Can you work these out from the drawing? Everything is in mm from the part's minimum corner. A direction names the side the tool comes from. Coordinates: 2 decimals unless noted, no trailing zeros. Loops run counter-clockwise (first coordinate to the right, second up) from the corner with the lowest first, then second, coordinate; pieces in that order, holes last. Notation, with made-up numbers: (41, -28) -> (63, -28) arc R27 cw to (63, 7) -> close; hole circle Ø8 at (-9.5, -9.5). An arc over 180 degrees is marked (long way). Use one line per item in the form item = value. Start each with the question number.
(1) Imagine slicing it at D-D (x = 37.5). List the corners of the cut face in (y, z) for me.
(2) Imagine slicing it at B-B (x = 47). List the corners of the cut face in (y, z) for me, plus the area to 3 significant figures.
(3) I need wall thicknesses on line 1 (Z direction, x = 37.5, y = 1.6); line 2 (Y direction, x = 37, z = 9.75); line 3 (Z direction, x = 40.5, y = 69). Which ranges of each line are inside material? Lowest first, please. Write a range as [from, to].
(4) On a 3-axis mill with a long thin cutter (end or side, diameter ignored), from which of +Z, -Z, +X, -X, +Y, -Y can I reach the whole of each face in a straight line? I mean the marked faces 1 and 2. Say none if no direction works.
(5) Imagine slicing it at A-A (z = 16.5). State how many separate pieces and enclosed holes the cut face has, plus the area to 3 significant figures.
(6) Imagine slicing it at C-C (y = 42.5). List the corners of the cut face in (x, z) for me, plus the area to 3 significant figures.
(7) I'm going to push flat-ended pins straight in: pin 1 (14.5 mm diameter, centred on x = 13.5, z = 18.5, fed in from +Y); pin 2 (2.5 mm diameter, centred on y = 92.5, z = 16.5, fed in from -X); pin 3 (10 mm diameter, centred on y = 31, z = 14, fed in from -X); pin 4 (10 mm diameter, centred on x = 30.5, y = 54.5, fed in from +Z). Where does each tip first touch, or does it pass through?
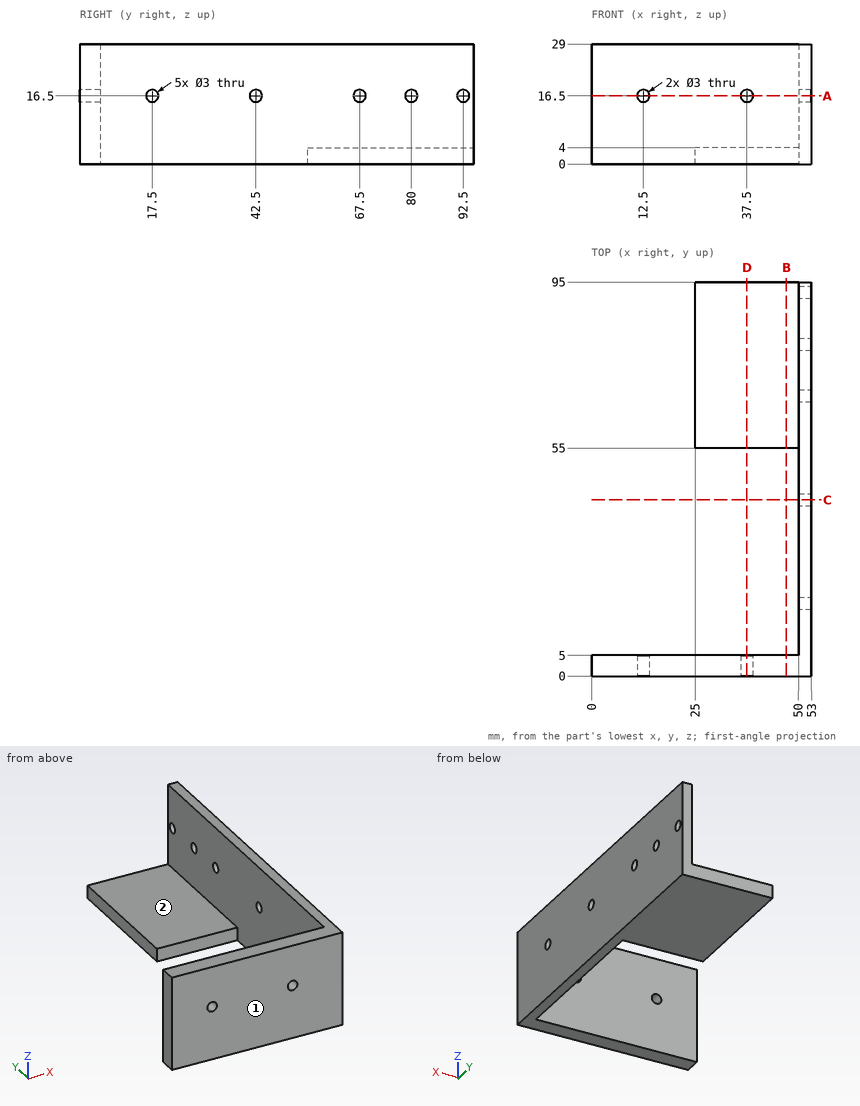
Worked out:
q1.outline = (0, 0) -> (5, 0) -> (5, 15) -> (0, 15) -> close; (0, 18) -> (5, 18) -> (5, 29) -> (0, 29) -> close; (55, 0) -> (95, 0) -> (95, 4) -> (55, 4) -> close
q2.outline = (0, 0) -> (5, 0) -> (5, 29) -> (0, 29) -> close; (55, 0) -> (95, 0) -> (95, 4) -> (55, 4) -> close
q2.area = 305 mm2
q3.line_1 = [0, 15], [18, 29]
q3.line_2 = [0, 5]
q3.line_3 = [0, 4]
q4.face_1 = +Z, -Z, +X, -X, -Y
q4.face_2 = +Z, -X, +Y
q5.separate_pieces = 8
q5.enclosed_holes = 0
q5.area = 460 mm2
q6.outline = (50, 0) -> (53, 0) -> (53, 15) -> (50, 15) -> close; (50, 18) -> (53, 18) -> (53, 29) -> (50, 29) -> close
q6.area = 78.0 mm2
q7.pin_1 = 5
q7.pin_2 = through
q7.pin_3 = 50
q7.pin_4 = 4
